```python
from build123d import *

# Parameters (mm, degrees)
F1_DEPTH = 25
F2_R     = 2.5
F3_DEPTH = 25
F4_R     = 4.99999
F5_F1_R  = 2.5
F5_F2_R  = 2.5
F5_F3_R  = 2.5


# Not quite as in the source:
# - a fillet or chamfer is up to 0.001 mm smaller than in the source, because OpenCascade refuses the exact size
# - a feature names something its author has since deleted; it is built from what else it names


with BuildPart() as f1:
    # F0 (on Top) → F1 (new body)
    with BuildSketch(Plane.XY):
        with BuildLine():
            ThreePointArc((11.9032669473, 15), (8.9743347592, 7.9289321881), (1.9032669473, 5))
            Line((1.9032669473, 5), (-64.0967330527, 5))
            ThreePointArc((-64.0967330527, 5), (-71.1678008646, 7.9289321881), (-74.0967330527, 15))
            Line((-74.0967330527, 15), (-79.0967330527, 15))
            Line((-79.0967330527, 15), (-79.0967330527, 10))
            ThreePointArc((-79.0967330527, 10), (-76.1678008646, 2.9289321881), (-69.0967330527, 0))
            Line((-69.0967330527, 0), (-49.3079621117, 0))
            Line((-49.3079621117, 0), (11.9032669473, -20.5484238273))
            Line((11.9032669473, -20.5484238273), (11.9032669473, -30.5484238273))
            Line((11.9032669473, -30.5484238273), (16.9032669473, -30.5484238273))
            Line((16.9032669473, -30.5484238273), (16.9032669473, 15))
            Line((16.9032669473, 15), (16.9032669473, 28.8165863603))
            Line((16.9032669473, 28.8165863603), (11.9032669473, 28.8165863603))
            Line((11.9032669473, 28.8165863603), (11.9032669473, 15))
        make_face()
        Polygon((-33.5967330527, 0), (11.9032669473, 0), (11.9032669473, -15.2742119136), align=None, mode=Mode.SUBTRACT)
    extrude(amount=F1_DEPTH)

    # F2 (on face) → F3 (cut)
    with BuildSketch(Plane.YZ.offset(16.9032669473)):
        with Locations((-25.5484238273, 12.5)):
            Circle(F2_R)
        with Locations((23.8165863603, 12.5)):
            Circle(F2_R)
    extrude(amount=-F3_DEPTH, mode=Mode.SUBTRACT)

    # F4 (radius 5 in the source; OpenCascade refuses exactly that, so slightly less here)
    f4_edges = [f1.edges().sort_by_distance(p)[0] for p in [
        (-79.096733, 15, 12.5),
    ]]
    fillet(f4_edges, radius=F4_R)

    # F5: fillet of radius 2.5 on 10 edges, made by hand

    # F5_f1
    f5_f1_edges = [f1.edges().sort_by_distance(p)[0] for p in [
        (-33.5967330527, 0, 12.5),
        (11.9032669473, 0, 12.5),
        (11.9032669473, -15.2742119136, 12.5),
        (-49.3079621117, 0, 12.5),
    ]]
    fillet(f5_f1_edges, radius=F5_F1_R)

    # F5_f2
    f5_f2_edges = [f1.edges().sort_by_distance(p)[0] for p in [
        (8.9743347592, 7.9289321881, 0),
        (-71.1678008646, 7.9289321881, 0),
        (-31.0967330527, 5, 0),
        (11.9032669473, 21.9082931802, 0),
    ]]
    fillet(f5_f2_edges, radius=F5_F2_R)

    # F5_f3
    f5_f3_edges = [f1.edges().sort_by_distance(p)[0] for p in [
        (11.9032669473, -7.148931772, 25),
        (-4.4453294203, 0, 25),
        (-20.7612174023, -2.0969217328, 25),
        (11.1710339003, -0.732233047, 25),
        (10.8628862029, -13.8275215518, 25),
    ]]
    fillet(f5_f3_edges, radius=F5_F3_R)


solid = f1.part
```
Can you work these out from the model? Positions are in its coordinate system, mm. A direction names the side the tool comes from. Give positions to 0.01 mm unless a question says otherwise; leave off trailing zeros. Loops run counter-clockwise (first coordinate to the right, second up) from the corner with the lowest first, then second, coordinate; pieces in that order, holes last. Notation, with made-up numbers: M 48.25,9 L 86.25,9 A18 ccw 86.25,44 Z; hole C 0.25,83.5 d6. An arc over 180 degrees is marked long. One line per question, with ' | ' between items. Start each with the question number.
Q1. If I drill on line 1 (X direction, y = -23, z = 8.5); line 2 (Y direction, x = -7, z = 14.75); line 3 (Y direction, x = -5, z = 9.25), over which ranges is the centre line in solid material (lowest first)? Write a range as from..to.
Q2. If we section it at C-C (x = -56): Please give me the cut outline in (y, z).
Q3. If we section it at A-A (z = 12.5): State how many separate pieces and enclosed holes the cut face has, plus the area to 3 significant figures.
Q4. For faces 4 (the flat face through (-60, 0, 12)), 5 (the flat face through (11.903, -7, 11)), 6 (the cylindrical face through (14.4, 25, 10.3)), 7 (the flat face through (-31, 5, 14)), 8 (the cylindrical face through (-5.66, -10.13, 24.25)), which set-ups out of +Z, -Z, +X, -X, +Y, -Y let a thin tool reach every point of the face, with its end or its side?
Q5. If we section it at D-D (x = -37.5): Please give me the cut outline in (y, z).
Q6. If we mould it in two halves opening along X, with no side actions, what happens to faces 1 (the flat face through (14, 28.817, 12)), 2 (the cylindrical face through (-77.593, 13.574, 12.675)), 3 (the cylindrical face through (-71.09, 7.85, 13.59))? For each: +X half, -X half, draft (parallel to the pull), parting line (faces both ways), or undercut.
Q7. For pin 1 Ø15 at (y, z) = (25, 16) entering from -X; pin 2 Ø4 at (x, y) = (2, -9) entering from +Z; pin 3 Ø10 at (x, z) = (-63, 4.5) entering from -Y; pin 4 Ø10 at (x, z) = (-9.5, 3) entering from +Y, each with a flat end and sliding along its axis, tell me the tip position at first contact or that it passes through.
Computed:
1) line 1: x = 11.9..16.9 | line 2: y = -14.2..-8.93, 0..5 | line 3: y = -14.87..-9.6, 0..5
2) outline: M 0,0 L 2.5,0 A2.5 ccw 5,2.5 L 5,25 L 0,25 Z
3) separate pieces: 3 | enclosed holes: 1 | area: 1,080 mm²
4) face 4: +Z, -Z, -X, -Y | face 5: +Z, -Z | face 6: +X, -X | face 7: +Z, -Z, +Y | face 8: +Z
5) outline: M -3.96,0 L 2.5,0 A2.5 ccw 5,2.5 L 5,25 L -3.96,25 Z
6) face 1: draft | face 2: -X half | face 3: undercut
7) pin 1: stops at x = 11.9 | pin 2: passes through | pin 3: stops at y = 0 | pin 4: stops at y = 5
